Verification items for the finished model (mm, model axes). Face numbers are marked on the shaded views. A direction names the side the tool comes from. Round coordinates to 2 decimals unless told otherwise and drop trailing zeros. Put each result on its own line as item: value.
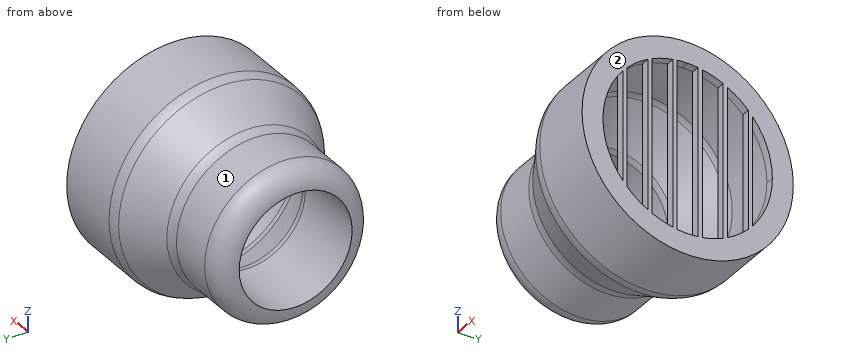
```python
from build123d import *

# Parameters (mm, degrees)
F2_R     = 25.25
F3_DEPTH = 2
F5_DEPTH = 2
F6_R     = 4.99999
F7_R     = 3


# Not quite as in the source:
# - a fillet or chamfer is up to 0.001 mm smaller than in the source, because OpenCascade refuses the exact size
# - a feature names something its author has since deleted; it is built from what else it names


with BuildPart() as f1:
    # F0 (on Top) → F1 (revolve)
    with BuildSketch(Plane.XY):
        Polygon((-18, 18.5), (-18, 13.5), (0, 13.5), (11.6913429511, 20.25), (25.1913429511, 20.25), (25.1913429511, 25.25), (10.3515969889, 25.25), (-1.3397459622, 18.5), align=None)
    revolve(axis=Axis((-8.7595172226, 0, 0), (1, 0, 0)))

    # F2 (on face) → F3 (join)
    with BuildSketch(Plane.YZ.offset(25.1913429511)):
        Circle(F2_R)
    extrude(amount=F3_DEPTH)

    # F4 (on face) → F5 (cut, through all)
    with BuildSketch(Plane.YZ.offset(27.1913429511)):
        with BuildLine():
            ThreePointArc((14.5, 14.1355049432), (12.1454310832, 16.2034256811), (9.5, 17.8833022678))
            Line((9.5, 17.8833022678), (9.5, -17.8833022678))
            ThreePointArc((9.5, -17.8833022678), (12.1454310832, -16.2034256811), (14.5, -14.1355049432))
            Line((14.5, -14.1355049432), (14.5, 14.1355049432))
        make_face()
        with BuildLine():
            ThreePointArc((8.5, 18.3796762757), (6.0508466769, 19.3248481105), (3.5, 19.9452375268))
            Line((3.5, 19.9452375268), (3.5, -19.9452375268))
            ThreePointArc((3.5, -19.9452375268), (6.0508466769, -19.3248481105), (8.5, -18.3796762757))
            Line((8.5, -18.3796762757), (8.5, 18.3796762757))
        make_face()
        with BuildLine():
            ThreePointArc((2.5, 20.0950864641), (1.2523975211, 20.2112345108), (0, 20.25))
            ThreePointArc((0, 20.25), (-1.2523975211, 20.2112345108), (-2.5, 20.0950864641))
            Line((-2.5, 20.0950864641), (-2.5, -20.0950864641))
            ThreePointArc((-2.5, -20.0950864641), (-1.2523975211, -20.2112345108), (0, -20.25))
            ThreePointArc((0, -20.25), (1.2523975211, -20.2112345108), (2.5, -20.0950864641))
            Line((2.5, -20.0950864641), (2.5, 20.0950864641))
        make_face()
        with BuildLine():
            Line((-3.5, -19.9452375268), (-3.5, 19.9452375268))
            ThreePointArc((-3.5, 19.9452375268), (-6.0508466769, 19.3248481105), (-8.5, 18.3796762757))
            Line((-8.5, 18.3796762757), (-8.5, -18.3796762757))
            ThreePointArc((-8.5, -18.3796762757), (-6.0508466769, -19.3248481105), (-3.5, -19.9452375268))
        make_face()
        with BuildLine():
            Line((-9.5, -17.8833022678), (-9.5, 17.8833022678))
            ThreePointArc((-9.5, 17.8833022678), (-12.1454310832, 16.2034256811), (-14.5, 14.1355049432))
            Line((-14.5, 14.1355049432), (-14.5, -14.1355049432))
            ThreePointArc((-14.5, -14.1355049432), (-12.1454310832, -16.2034256811), (-9.5, -17.8833022678))
        make_face()
        with BuildLine():
            Line((-15.5, -13.0312125299), (-15.5, 13.0312125299))
            ThreePointArc((-15.5, 13.0312125299), (-20.25, 0), (-15.5, -13.0312125299))
        make_face()
        with BuildLine():
            ThreePointArc((20.25, 0), (19.0254763409, 6.9349657533), (15.5, 13.0312125299))
            Line((15.5, 13.0312125299), (15.5, -13.0312125299))
            ThreePointArc((15.5, -13.0312125299), (19.0254763409, -6.9349657533), (20.25, 0))
        make_face()
    extrude(amount=-F5_DEPTH, mode=Mode.SUBTRACT)

    # F6 (radius 5 in the source; OpenCascade refuses exactly that, so slightly less here)
    f6_edges = [f1.edges().sort_by_distance(p)[0] for p in [
        (-18, -18.5, 0),
        (-1.339746, -18.5, 0),
        (10.351597, -25.25, 0),
    ]]
    fillet(f6_edges, radius=F6_R)

    # F7
    f7_edges = [f1.edges().sort_by_distance(p)[0] for p in [
        (11.691343, -20.25, 0),
        (0, -13.5, 0),
    ]]
    fillet(f7_edges, radius=F7_R)


solid = f1.part
```
Item 1: Material ranges on line 1 along Z through (x, y) = (-14, 0); line 2 along Y through (x, z) = (17, 0); line 3 along Y through (x, z) = (-4.5, 0), recorded low to high.
Geometry check:
line 1: -18.4 to -13.5, 13.5 to 18.4
line 2: -25.25 to -20.25, 20.25 to 25.25
line 3: -18.5 to -13.5, 13.5 to 18.5
Item 2: Depth check by flat-ended pin: pin 1 Ø1 at (x, y) = (13, -17.5) entering from +Z; pin 2 Ø5 at (x, z) = (-1.5, -9.5) entering from -Y; pin 3 Ø1.5 at (x, z) = (15.5, -2.5) entering from -Y. Enter the tip coordinate at first touch or a pass-through.
Geometry check:
pin 1: z = 18.67
pin 2: y = -17.85
pin 3: y = -25.19
Item 3: Tool access check on the marked faces 1 and 2. Record the directions out of +Z, -Z, +X, -X, +Y, -Y that give a thin tool (end or side, any length) a straight path to the whole face; none if there is none.
Geometry check:
face 1: -X
face 2: +Z, -Z, +X, +Y, -Y
